For this review, take the finished solid that the model builds, in its own axes (mm). Face numbers are marked on the shaded views. Give positions to 0.01 mm unless a question says otherwise; leave off trailing zeros. Loops run counter-clockwise (first coordinate to the right, second up) from the corner with the lowest first, then second, coordinate; pieces in that order, holes last.
```python
from build123d import *

# Parameters (mm, degrees)
AUFSATZ_LINEAR_AUSTRAGEN1_DEPTH = 50
SKIZZE2_W                       = 6.907618634
SKIZZE2_H                       = 20
AUFSATZ_LINEAR_AUSTRAGEN2_DEPTH = 10
AUFSATZ_LINEAR_START            = -50
SKIZZE2_2_W                     = 6.907618634
SKIZZE2_2_H                     = 20
AUFSATZ_LINEAR_AUSTRAGEN3_DEPTH = 10
FASE1_SIZE                      = 0.75
FASE1_SIZE_2                    = 0.55222801
SKIZZE3_R                       = 2.3
SCHNITT_LINEAR_AUSTRAGEN1_DEPTH = 10
VERRUNDUNG1_R                   = 2
FASE2_SIZE                      = 0.6


with BuildPart() as part:
    # Skizze1 → Aufsatz-Linear austragen1 (new body)
    with BuildSketch(Plane.XY):
        Polygon((0, 0), (0, 10), (-1.407618634, 10), (-6.907618634, 0), align=None)
    extrude(amount=AUFSATZ_LINEAR_AUSTRAGEN1_DEPTH)

    # Skizze2 → Aufsatz-Linear austragen2 (add)
    with BuildSketch(Plane.XY.offset(50)):
        with Locations((-3.453809317, 10)):
            Rectangle(SKIZZE2_W, SKIZZE2_H)
    extrude(amount=AUFSATZ_LINEAR_AUSTRAGEN2_DEPTH)

    # Skizze2<2> → Aufsatz-Linear austragen3 (add)
    with BuildSketch(Plane.XY.offset(50).offset(AUFSATZ_LINEAR_START)):
        with Locations((-3.453809317, 10)):
            Rectangle(SKIZZE2_2_W, SKIZZE2_2_H)
    extrude(amount=-AUFSATZ_LINEAR_AUSTRAGEN3_DEPTH)

    # Fase1
    # the kernel refuses this chamfer: 0.75, 0.55222801 mm, written as the material it takes off along each edge
    with BuildSketch(Plane(origin=(-6.907618634, 0, 50), x_dir=(-0.027495876610586778, 0.9996219169112968, 0), z_dir=(0, 0, 1))) as fase1_piece_1:
        Polygon((FASE1_SIZE * 0.999621916911, -FASE1_SIZE * 0.0274958766106), (-FASE1_SIZE * 0.0274958766106, -FASE1_SIZE * 0.999621916911), (0, 0), align=None)
    extrude(amount=11.928762241, mode=Mode.SUBTRACT)
    with BuildSketch(Plane(origin=(-6.907618634, 0, 0), x_dir=(-0.027495876610586778, 0.9996219169112968, 0), z_dir=(0, 0, -1))) as fase1_piece_2:
        Polygon((FASE1_SIZE * 0.999621916911, FASE1_SIZE * 0.0274958766106), (-FASE1_SIZE * 0.0274958766106, FASE1_SIZE * 0.999621916911), (0, 0), align=None)
    extrude(amount=11.928762241, mode=Mode.SUBTRACT)
    with BuildSketch(Plane(origin=(-6.907618634, 0, 0), x_dir=(0.436311778339264, 0.8997955501570503, 0), z_dir=(0, 0, 1))) as fase1_piece_3:
        Polygon((FASE1_SIZE_2 * 0.998682002669, -FASE1_SIZE_2 * 0.0513250252757), (FASE1_SIZE * 0.436311778339, -FASE1_SIZE * 0.899795550157), (0, 0), align=None)
    extrude(amount=50, mode=Mode.SUBTRACT)

    # Skizze3 → Schnitt-Linear austragen1 (cut)
    with BuildSketch(Plane.ZY.offset(6.907618634)):
        with Locations(Location((-5, 10, 0), (0, 0, 270))):
            Circle(SKIZZE3_R)
        with Locations((55, 10)):
            Circle(SKIZZE3_R)
    extrude(amount=-SCHNITT_LINEAR_AUSTRAGEN1_DEPTH, mode=Mode.SUBTRACT)

    # Verrundung1
    verrundung1_edges = [part.edges().sort_by_distance(p)[0] for p in [
        (-3.078809317, 0, -10),
        (-3.078809317, 0, 60),
        (-3.453809317, 20, 60),
        (-3.453809317, 20, 50),
        (-3.453809317, 20, 0),
        (-3.453809317, 20, -10),
    ]]
    fillet(verrundung1_edges, radius=VERRUNDUNG1_R)

    # Fase2
    fase2_edges = [part.edges().sort_by_distance(p)[0] for p in [
        (0, 0, 25),
        (0, 0.585786438, 59.414213562),
        (0, 0.585786438, -9.414213562),
        (0, 10, 60),
        (0, 10, -10),
        (0, 19.414213562, 59.414213562),
        (0, 19.414213562, -9.414213562),
        (0, 20, 55),
        (0, 20, -5),
        (0, 19.414213562, 50.585786438),
        (0, 19.414213562, -0.585786438),
        (0, 14, 50),
        (0, 14, 0),
    ]]
    chamfer(fase2_edges, length=FASE2_SIZE)
    fase2_2_edges = [part.edges().sort_by_distance(p)[0] for p in [
        (0, 10, 25),
    ]]
    chamfer(fase2_2_edges, length=FASE2_SIZE)
    fase2_3_edges = [part.edges().sort_by_distance(p)[0] for p in [
        (0, 10, 52.7),
    ]]
    chamfer(fase2_3_edges, length=FASE2_SIZE)
    fase2_4_edges = [part.edges().sort_by_distance(p)[0] for p in [
        (0, 12.3, -5),
    ]]
    chamfer(fase2_4_edges, length=FASE2_SIZE)
    fase2_5_edges = [part.edges().sort_by_distance(p)[0] for p in [
        (-6.907618634, 1.337617557, 59.887127314),
        (-6.907618634, 10, 60),
        (-6.907618634, 19.414213562, 59.414213562),
        (-6.907618634, 20, 55),
        (-6.907618634, 19.414213562, 50.585786438),
        (-6.907618634, 9.375, 50),
    ]]
    chamfer(fase2_5_edges, length=FASE2_SIZE)
    fase2_6_edges = [part.edges().sort_by_distance(p)[0] for p in [
        (-6.907618634, 1.337617557, -9.887127314),
        (-6.907618634, 10, -10),
        (-6.907618634, 19.414213562, -9.414213562),
        (-6.907618634, 20, -5),
        (-6.907618634, 19.414213562, -0.585786438),
        (-6.907618634, 9.375, 0),
    ]]
    chamfer(fase2_6_edges, length=FASE2_SIZE)
    fase2_7_edges = [part.edges().sort_by_distance(p)[0] for p in [
        (-6.907618634, 10, 52.7),
    ]]
    chamfer(fase2_7_edges, length=FASE2_SIZE)
    fase2_8_edges = [part.edges().sort_by_distance(p)[0] for p in [
        (-6.907618634, 12.3, -5),
    ]]
    chamfer(fase2_8_edges, length=FASE2_SIZE)


solid = part.part
```
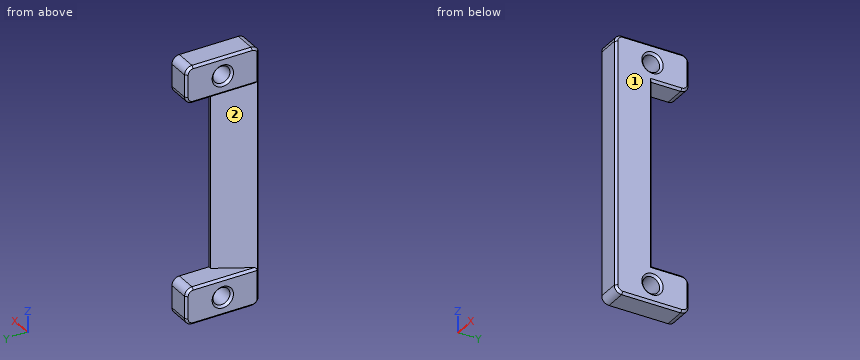
Q1. Consider section D-D on x = -5.5. Give the boundary of the cut face in (y, z).
Answers:
outline: (0, -8) arc R2 ccw to (2, -10) - (18, -10) arc R2 ccw to (20, -8) - (20, -2) arc R2 ccw to (18, 0) - (2.56, 0) - (2.56, 50) - (18, 50) arc R2 ccw to (20, 52) - (20, 58) arc R2 ccw to (18, 60) - (2, 60) arc R2 ccw to (0, 58) - close; hole circle Ø4.6 at (10, -5); hole circle Ø4.6 at (10, 55)
Q2. Consider section A-A on z = -5. Give the boundary of the cut face in (x, y).
Answers:
outline: (-6.91, 0.75) - (-6.16, 0) - (-0.6, 0) - (0, 0.6) - (0, 7.1) - (-0.6, 7.7) - (-6.31, 7.7) - (-6.91, 7.1) - close; (-6.91, 12.9) - (-6.31, 12.3) - (-0.6, 12.3) - (0, 12.9) - (0, 19.4) - (-0.6, 20) - (-6.31, 20) - (-6.91, 19.4) - close
Q3. For pin 1 Ø2 at (x, z) = (-1.5, 37.5) entering from +Y; pin 2 Ø12 at (y, z) = (15, 27) entering from +X; pin 3 Ø1 at (x, z) = (-4.5, 17.5) entering from +Y, all flat-tipped, find the tip position at first contact; note any pin that passes through.
Answers:
pin 1: stops at y = 10
pin 2: stops at x = 0
pin 3: stops at y = 5.29
Q4. Consider section B-B on y = 15.25. Give the boundary of the cut face in (x, z).
Answers:
outline: (-6.91, -9.4) - (-6.31, -10) - (-0.6, -10) - (0, -9.4) - (0, -0.6) - (-0.6, 0) - (-6.31, 0) - (-6.91, -0.6) - close; (-6.91, 50.6) - (-6.31, 50) - (-0.6, 50) - (0, 50.6) - (0, 59.4) - (-0.6, 60) - (-6.31, 60) - (-6.91, 59.4) - close
Q5. Mouldability with a two-part tool opening along X and no side actions: class the marked faces 1 and 2 as +X half, -X half, draft (parallel to the pull), parting line (faces both ways), or undercut.
Answers:
face 1: +X half
face 2: -X half
Q6. Consider section C-C on z = 2.5. Give the boundary of the cut face in (x, y).
Answers:
outline: (-6.64, 0.48) - (-6.16, 0) - (-0.6, 0) - (0, 0.6) - (0, 9.4) - (-0.6, 10) - (-1.41, 10) - close
Q7. For probe 1 along Y at (x, z) = (-3.7, 55); probe 2 along Z at (x, y) = (-4.5, 11.5); probe 3 along Z at (x, y) = (-5.5, 9.5) (3 decimals), list the stretches that pass through material, from the lowest coordinate up.
Answers:
probe 1: y = 0 to 7.7, 12.3 to 20
probe 2: z = -10 to -6.74, -3.26 to 0, 50 to 53.26, 56.74 to 60
probe 3: z = -10 to -7.245, -2.755 to 0, 50 to 52.755, 57.245 to 60
